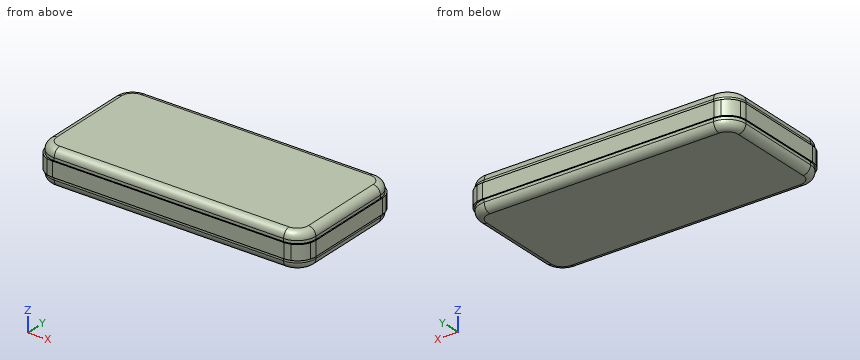
from build123d import *

# Parameters (mm, degrees)
ESQUISSE1_W        = 144
ESQUISSE1_H        = 67
BOSS_EXTRU_1_DEPTH = 9.5
CONG_2_R           = 10
CONG_1_R           = 4
ESQUISSE3_W        = 145.2
ESQUISSE3_H        = 68.2
ESQUISSE3_W_2      = 144
ESQUISSE3_H_2      = 67
BOSS_EXTRU_2_DEPTH = 4
CONG_3_START       = -4
CONG_3_DEPTH       = 8
CONG_3_2_DEPTH     = 8


with BuildPart() as part:
    # Esquisse1 → Boss.-Extru.1 (new, symmetric)
    with BuildSketch(Plane.XY):
        Rectangle(ESQUISSE1_W, ESQUISSE1_H)
    extrude(amount=BOSS_EXTRU_1_DEPTH, both=True)

    # Congé2
    cong_2_edges = [part.edges().sort_by_distance(p)[0] for p in [
        (-72, 33.5, 0),
        (72, 33.5, 0),
        (72, -33.5, 0),
        (-72, -33.5, 0),
    ]]
    fillet(cong_2_edges, radius=CONG_2_R)

    # Congé1
    cong_1_edges = [part.edges().sort_by_distance(p)[0] for p in [
        (0, -33.5, -9.5),
        (0, -33.5, 9.5),
        (-72, 0, -9.5),
        (0, 33.5, -9.5),
        (72, 0, -9.5),
        (69.071067812, 30.571067812, -9.5),
        (69.071067812, -30.571067812, -9.5),
        (-69.071067812, 30.571067812, -9.5),
        (-69.071067812, -30.571067812, -9.5),
        (-72, 0, 9.5),
        (72, 0, 9.5),
        (0, 33.5, 9.5),
        (69.071067812, 30.571067812, 9.5),
        (69.071067812, -30.571067812, 9.5),
        (-69.071067812, 30.571067812, 9.5),
        (-69.071067812, -30.571067812, 9.5),
    ]]
    fillet(cong_1_edges, radius=CONG_1_R)

    # Esquisse3 → Boss.-Extru.2 (add, symmetric)
    with BuildSketch(Plane.XY):
        Rectangle(ESQUISSE3_W, ESQUISSE3_H)
        Rectangle(ESQUISSE3_W_2, ESQUISSE3_H_2, mode=Mode.SUBTRACT)
    extrude(amount=BOSS_EXTRU_2_DEPTH, both=True)

    # Congé3: read off the stored shape, not the designer's step
    # Congé3 outline → Congé3 (cut)
    with BuildSketch(Plane.XY.offset(CONG_3_START)):
        with BuildLine():
            Line((-72.6, 34.1), (-72.6, 24.1))
            ThreePointArc((-72.6, 24.1), (-72.448857802, 25.832050808), (-72, 27.511744422))
            Line((-72, 27.511744422), (-72, 33.5))
            Line((-72, 33.5), (-66.011744422, 33.5))
            ThreePointArc((-66.011744422, 33.5), (-64.332050808, 33.948857802), (-62.6, 34.1))
            Line((-62.6, 34.1), (-72.6, 34.1))
        make_face()
        with BuildLine():
            ThreePointArc((-72, -27.511744422), (-72.448857802, -25.832050808), (-72.6, -24.1))
            Line((-72.6, -24.1), (-72.6, -34.1))
            Line((-72.6, -34.1), (-62.6, -34.1))
            ThreePointArc((-62.6, -34.1), (-64.332050808, -33.948857802), (-66.011744422, -33.5))
            Line((-66.011744422, -33.5), (-72, -33.5))
            Line((-72, -33.5), (-72, -27.511744422))
        make_face()
        with BuildLine():
            Line((72.6, 34.1), (62.6, 34.1))
            ThreePointArc((62.6, 34.1), (64.332050808, 33.948857802), (66.011744422, 33.5))
            Line((66.011744422, 33.5), (72, 33.5))
            Line((72, 33.5), (72, 27.511744422))
            ThreePointArc((72, 27.511744422), (72.448857802, 25.832050808), (72.6, 24.1))
            Line((72.6, 24.1), (72.6, 34.1))
        make_face()
        with BuildLine():
            ThreePointArc((66.011744422, -33.5), (64.332050808, -33.948857802), (62.6, -34.1))
            Line((62.6, -34.1), (72.6, -34.1))
            Line((72.6, -34.1), (72.6, -24.1))
            ThreePointArc((72.6, -24.1), (72.448857802, -25.832050808), (72, -27.511744422))
            Line((72, -27.511744422), (72, -33.5))
            Line((72, -33.5), (66.011744422, -33.5))
        make_face()
    extrude(amount=CONG_3_DEPTH, mode=Mode.SUBTRACT)

    # Cong_3 2 outline → Cong_3 2 (add)
    with BuildSketch(Plane.XY.offset(CONG_3_START)):
        with BuildLine():
            ThreePointArc((-66.011744422, 33.5), (-69.671067812, 31.171067812), (-72, 27.511744422))
            Line((-72, 27.511744422), (-72, 23.5))
            ThreePointArc((-72, 23.5), (-69.071067812, 30.571067812), (-62, 33.5))
            Line((-62, 33.5), (-66.011744422, 33.5))
        make_face()
        with BuildLine():
            Line((-72, -23.5), (-72, -27.511744422))
            ThreePointArc((-72, -27.511744422), (-69.671067812, -31.171067812), (-66.011744422, -33.5))
            Line((-66.011744422, -33.5), (-62, -33.5))
            ThreePointArc((-62, -33.5), (-69.071067812, -30.571067812), (-72, -23.5))
        make_face()
        with BuildLine():
            ThreePointArc((72, 27.511744422), (69.671067812, 31.171067812), (66.011744422, 33.5))
            Line((66.011744422, 33.5), (62, 33.5))
            ThreePointArc((62, 33.5), (69.071067812, 30.571067812), (72, 23.5))
            Line((72, 23.5), (72, 27.511744422))
        make_face()
        with BuildLine():
            Line((62, -33.5), (66.011744422, -33.5))
            ThreePointArc((66.011744422, -33.5), (69.671067812, -31.171067812), (72, -27.511744422))
            Line((72, -27.511744422), (72, -23.5))
            ThreePointArc((72, -23.5), (69.071067812, -30.571067812), (62, -33.5))
        make_face()
    extrude(amount=CONG_3_2_DEPTH)


solid = part.part
The model under review builds one solid part; all positions refer to its coordinate system, in mm. Coordinates: 2 decimals unless noted, no trailing zeros. Write each loop counter-clockwise with the first axis right and the second up, starting at its lowest first coordinate (ties: lowest second). Pieces come first, ordered by that corner, then holes. Notation, with made-up numbers: (68.5, -31) - (91.5, -31) arc R29 ccw to (91.5, -9) - close; hole circle Ø8 at (16, 27.5). An arc over 180 degrees is marked (long way). Answer as a JSON object with one key per item and string values. Group by question number.
1. Clearance check with flat-ended pins moving along their axes: pin 1 Ø0.8 at (x, z) = (-0.5, -4.5) entering from +Y; pin 2 Ø0.8 at (y, z) = (-4, 4.5) entering from +X; pin 3 Ø0.5 at (y, z) = (-10, -4.5) entering from -X. State where each tip first meets the part, or that it passes through.
2. Add section B-B (z = -7). Give the boundary of the cut face in (x, y), plus the area to 3 significant figures.
3. To check wall thickness, follow probe 1 along Y at (x, z) = (14, 4.25); probe 2 along X at (y, z) = (-9.5, 4.25); probe 3 along Y at (x, z) = (63, -0.5). State the ranges of each line that lie inside material, in increasing order.
4. Add section A-A (x = -7). Give the boundary of the cut face in (y, z), plus the area to 3 significant figures.
Findings:
{
 "1": {"pin 1": "y = 33.5", "pin 2": "x = 72", "pin 3": "x = -72"},
 "2": {"outline": "(-71.71, -23.5) arc R9.71 ccw to (-62, -33.21) - (62, -33.21) arc R9.71 ccw to (71.71, -23.5) - (71.71, 23.5) arc R9.71 ccw to (62, 33.21) - (-62, 33.21) arc R9.71 ccw to (-71.71, 23.5) - close", "area": "9,440 mm²"},
 "3": {"probe 1": "-33.5 to 33.5", "probe 2": "-72 to 72", "probe 3": "-34.09 to 34.09"},
 "4": {"outline": "(-34.1, -4) - (-33.5, -4) - (-33.5, -5.5) arc R4 ccw to (-29.5, -9.5) - (29.5, -9.5) arc R4 ccw to (33.5, -5.5) - (33.5, -4) - (34.1, -4) - (34.1, 4) - (33.5, 4) - (33.5, 5.5) arc R4 ccw to (29.5, 9.5) - (-29.5, 9.5) arc R4 ccw to (-33.5, 5.5) - (-33.5, 4) - (-34.1, 4) - close", "area": "1,270 mm²"}
}
